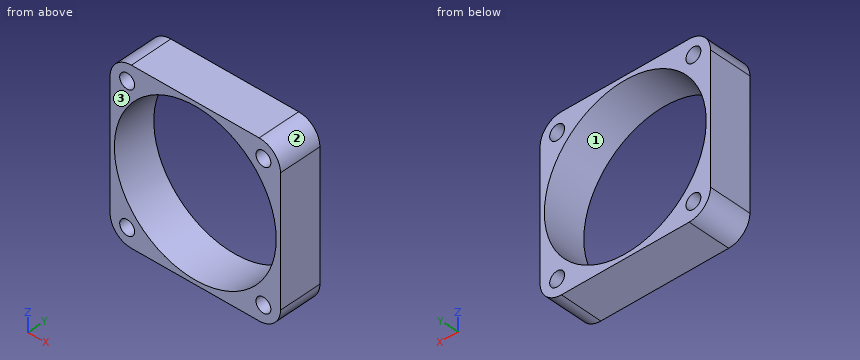
```python
from build123d import *

# Parameters (mm, degrees)
F0_W     = 40
F0_H     = 40
F0_R     = 1.75
F0_R_2   = 19
F1_DEPTH = 10
F2_R     = 5


with BuildPart() as f1:
    # F0 (on Front) → F1 (new body)
    with BuildSketch(Plane.XZ):
        Rectangle(F0_W, F0_H)
        with Locations((-16, -16)):
            Circle(F0_R, mode=Mode.SUBTRACT)
        with Locations((16, -16)):
            Circle(F0_R, mode=Mode.SUBTRACT)
        with Locations((-16, 16)):
            Circle(F0_R, mode=Mode.SUBTRACT)
        Circle(F0_R_2, mode=Mode.SUBTRACT)
        with Locations((16, 16)):
            Circle(F0_R, mode=Mode.SUBTRACT)
    extrude(amount=F1_DEPTH)

    # F2
    f2_edges = [f1.edges().sort_by_distance(p)[0] for p in [
        (-20, -5, 20),
        (20, -5, 20),
        (20, -5, -20),
        (-20, -5, -20),
    ]]
    fillet(f2_edges, radius=F2_R)


solid = f1.part
```
CAD build for the part. Positions are in the model's coordinates, mm. Face numbers are marked on the shaded views. Coordinates: 2 decimals unless noted, no trailing zeros. Order: outer loops, then holes, each group sorted by start corner. A loop starts at its lowest first (then second) coordinate and runs counter-clockwise, first axis right, second up. Notation, with made-up numbers: (52.25, 87.5) - (97.25, 87.5) arc R9 cw to (97.25, 104.5) - close; hole circle Ø8 at (68, 2.5). An arc over 180 degrees is marked (long way). Use a Markdown table: item, result. Add a question column.
(1) Saw through at D-D (x = -16). Give the cut face in (y, z), then the cut area to 3 significant figures.
(2) Saw through at B-B (x = 0). Give the cut face in (y, z), then the cut area to 3 significant figures.
(3) Pull direction Z, two halves, no side cores. Call the marked faces 1, 2 and 3: +Z half, -Z half, draft (parallel to the pull), parting line (faces both ways), or undercut.
(4) Saw through at A-A (y = -2.25). Give the cut face in (x, z).
(5) Saw through at C-C (z = -4). Give the cut face in (x, y), then the cut area to 3 significant figures.
(6) Drill centre lines: line 1 along Z through (x, y) = (16, -2.75); line 2 along X through (y, z) = (-7, -16.5); line 3 along Z through (x, y) = (-0.5, -8.25). Where is each one in solid material? Low to high. Write a range as [from, to].
Solved:
| question | item | result |
|---|---|---|
| 1 | outline | (-10, -19.9) - (0, -19.9) - (0, -17.75) - (-10, -17.75) - close; (-10, -14.25) - (0, -14.25) - (0, -10.25) - (-10, -10.25) - close; (-10, 10.25) - (0, 10.25) - (0, 14.25) - (-10, 14.25) - close; (-10, 17.75) - (0, 17.75) - (0, 19.9) - (-10, 19.9) - close |
| 1 | area | 123 mm² |
| 2 | outline | (-10, -20) - (0, -20) - (0, -19) - (-10, -19) - close; (-10, 19) - (0, 19) - (0, 20) - (-10, 20) - close |
| 2 | area | 20.0 mm² |
| 3 | face 1 | undercut |
| 3 | face 2 | +Z half |
| 3 | face 3 | draft |
| 4 | outline | (-20, -15) arc R5 ccw to (-15, -20) - (15, -20) arc R5 ccw to (20, -15) - (20, 15) arc R5 ccw to (15, 20) - (-15, 20) arc R5 ccw to (-20, 15) - close; hole circle Ø38 at (0, 0); hole circle Ø3.5 at (-16, -16); hole circle Ø3.5 at (-16, 16); hole circle Ø3.5 at (16, -16); hole circle Ø3.5 at (16, 16) |
| 5 | outline | (-20, -10) - (-18.57, -10) - (-18.57, 0) - (-20, 0) - close; (18.57, -10) - (20, -10) - (20, 0) - (18.57, 0) - close |
| 5 | area | 28.5 mm² |
| 6 | line 1 | z = [-19.9, -17.75], [-14.25, -10.25], [10.25, 14.25], [17.75, 19.9] |
| 6 | line 2 | x = [-19.77, -17.68], [-14.32, -9.42], [9.42, 14.32], [17.68, 19.77] |
| 6 | line 3 | z = [-20, -18.99], [18.99, 20] |
